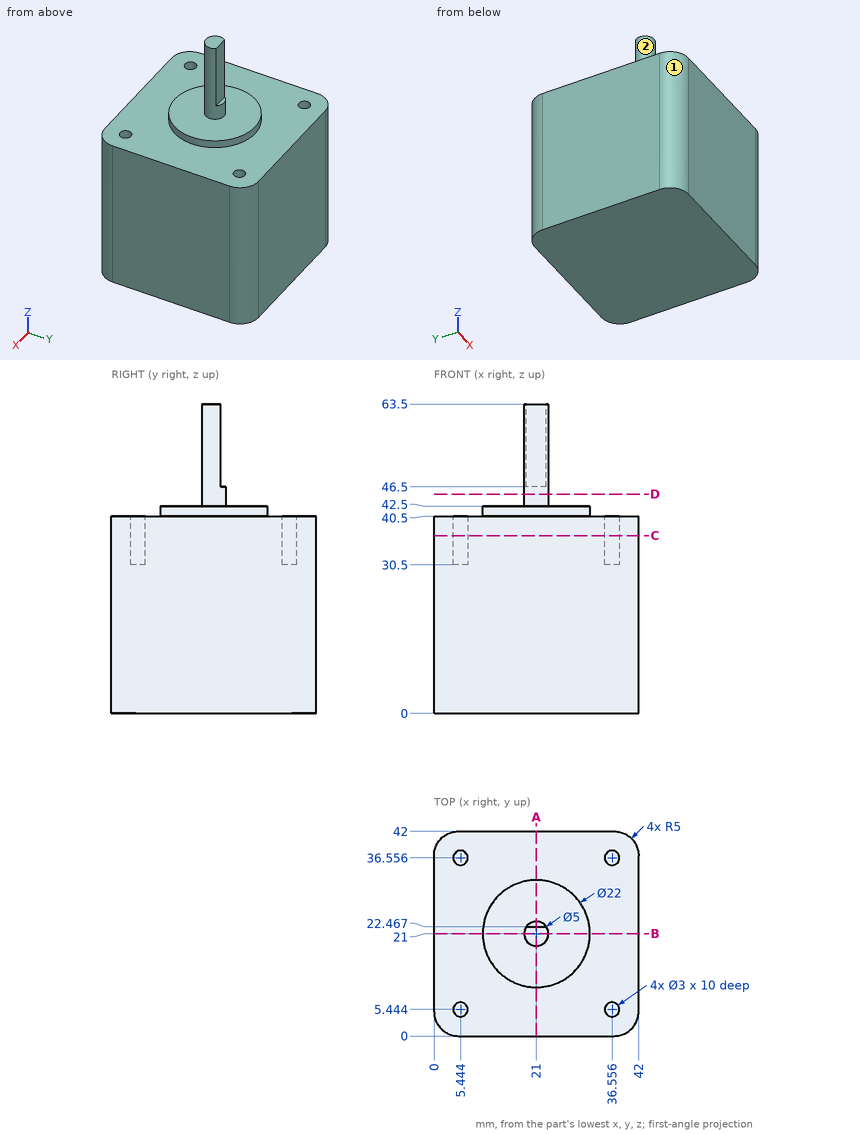
Study the drawing (mm; zero at the part's minimum x, y, z) and answer. A direction names the side the tool comes from. Coordinates: 2 decimals unless noted, no trailing zeros. Loops run counter-clockwise (first coordinate to the right, second up) from the corner with the lowest first, then second, coordinate; pieces in that order, holes last. Notation, with made-up numbers: M 16,-5 L 40,-5 A26 cw 40,34 Z; hole C -10,62.5 d9. An arc over 180 degrees is marked long. Answer in a Markdown table with one row per item.
1) Find section D-D (z = 45). Determine the outline of the cut face in (x, y).
Answers below:
| item | result |
|---|---|
| outline | C 21,21 d5 |
2) Which of the six approach directions +Z, -Z, +X, -X, +Y, -Y give full straight-line access (tool end or side, diameter ignored) to the marked faces 1 and 2?
Answers below:
| item | result |
|---|---|
| face 1 | +Z, -Z, -X, -Y |
| face 2 | +Z |
3) Find section B-B (y = 21). Determine the outline of the cut face in (x, z).
Answers below:
| item | result |
|---|---|
| outline | M 0,0 L 42,0 L 42,40.5 L 32,40.5 L 32,42.5 L 23.5,42.5 L 23.5,63.5 L 18.5,63.5 L 18.5,42.5 L 10,42.5 L 10,40.5 L 0,40.5 Z |
4) Given pin 1 (8 mm diameter, centred on x = 35.5, z = 25.5, fed in from -Y); pin 2 (1.5 mm diameter, centred on x = 37, y = 36.5, fed in from +Z); pin 3 (2.5 mm diameter, centred on x = 36.5, y = 5, fed in from +Z); pin 4 (3 mm diameter, centred on y = 25, z = 49.5, fed in from -X), each flat-ended and moving along its own axis, determine where each tip first touches the part or whether it passes through.
Answers below:
| item | result |
|---|---|
| pin 1 | y = 0 |
| pin 2 | z = 30.5 |
| pin 3 | z = 40.5 |
| pin 4 | through |
5) Find section C-C (z = 36.5). Determine the outline of the cut face in (x, y).
Answers below:
| item | result |
|---|---|
| outline | M 0,5 A5 ccw 5,0 L 37,0 A5 ccw 42,5 L 42,37 A5 ccw 37,42 L 5,42 A5 ccw 0,37 Z; hole C 5.44,5.44 d3; hole C 5.44,36.56 d3; hole C 36.56,5.44 d3; hole C 36.56,36.56 d3 |
6) Find section A-A (x = 21). Determine the outline of the cut face in (y, z).
Answers below:
| item | result |
|---|---|
| outline | M 0,0 L 42,0 L 42,40.5 L 32,40.5 L 32,42.5 L 23.5,42.5 L 23.5,46.5 L 22.47,46.5 L 22.47,63.5 L 18.5,63.5 L 18.5,42.5 L 10,42.5 L 10,40.5 L 0,40.5 Z |
7) Find the intervals of material crossed by probe 1 along Z at (x, y) = (22, 3); probe 2 along Z at (x, y) = (23, 10.5), in increasing order.
Answers below:
| item | result |
|---|---|
| probe 1 | 0 to 40.5 |
| probe 2 | 0 to 42.5 |
